Work out the finished part from the listing and answer in its coordinate system (mm). A direction names the side the tool comes from. Round coordinates to 2 decimals unless told otherwise and drop trailing zeros. Order: outer loops, then holes, each group sorted by start corner. A loop starts at its lowest first (then second) coordinate and runs counter-clockwise, first axis right, second up. Notation, with made-up numbers: M 63.25,-4 L 101.25,-4 A28 ccw 101.25,15 Z; hole C 77.5,28 d7. An arc over 180 degrees is marked long. Return JSON: item names as keys, results as strings.
from build123d import *

# Parameters (mm, degrees)
SKETCH1_R           = 3
BOSS_EXTRUDE1_DEPTH = 0.5
SKETCH2_R           = 2
BOSS_EXTRUDE2_DEPTH = 5
FILLET1_R           = 0.2


with BuildPart() as part:
    # Sketch1 → Boss-Extrude1 (new, symmetric)
    with BuildSketch(Plane.XY):
        Circle(SKETCH1_R)
    extrude(amount=BOSS_EXTRUDE1_DEPTH, both=True)

    # Sketch2 → Boss-Extrude2 (add)
    with BuildSketch(Plane.XY.offset(0.5)):
        Circle(SKETCH2_R)
    extrude(amount=BOSS_EXTRUDE2_DEPTH)

    # Fillet1
    fillet1_edges = [part.edges().sort_by_distance(p)[0] for p in [
        (-3, 0, -0.5),
        (-3, 0, 0.5),
        (-2, 0, 0.5),
        (-2, 0, 5.5),
    ]]
    fillet(fillet1_edges, radius=FILLET1_R)


solid = part.part
Item 1: Each of these flat-tipped pins is pushed along its axis until it touches: pin 1 (1.5 mm diameter, centred on x = 0.5, z = 2, fed in from -Y); pin 2 (1.5 mm diameter, centred on y = -1.5, z = 4.5, fed in from +X); pin 3 (1.5 mm diameter, centred on y = 1, z = 4.5, fed in from -X). Where does it stop, or does it pass through?
Output:
{"pin 1": "stops at y = -2", "pin 2": "stops at x = 1.85", "pin 3": "stops at x = -1.98"}
Item 2: Consider line 1 along Z through (x, y) = (-2.25, 0.5); line 2 along Y through (x, z) = (0, 3.7); line 3 along X through (y, z) = (1.25, 0.7). Determine where each line is inside the solid, lowest interval first. Write a range as [from, to].
Output:
{"line 1": "z = [-0.5, 0.5]", "line 2": "y = [-2, 2]", "line 3": "x = [-1.56, 1.56]"}
Item 3: Find section C-C (z = 1.7). Determine the outline of the cut face in (x, y).
Output:
{"outline": "C 0,0 d4"}
Item 4: Which of the six approach directions +Z, -Z, +X, -X, +Y, -Y give full straight-line access (tool end or side, diameter ignored) to faces 1 (the cylindrical face through (-3, 0, 0)), 2 (the cylindrical face through (0, -2, 3))?
Output:
{"face 1": "+Z, -Z", "face 2": "+Z"}
Item 5: Find section A-A (y = 0). Determine the outline of the cut face in (x, z).
Output:
{"outline": "M -3,-0.3 A0.2 ccw -2.8,-0.5 L 2.8,-0.5 A0.2 ccw 3,-0.3 L 3,0.3 A0.2 ccw 2.8,0.5 L 2.2,0.5 A0.2 cw 2,0.7 L 2,5.3 A0.2 ccw 1.8,5.5 L -1.8,5.5 A0.2 ccw -2,5.3 L -2,0.7 A0.2 cw -2.2,0.5 L -2.8,0.5 A0.2 ccw -3,0.3 Z"}
